Check sheet for the drawn part. Datum: minimum x, y, z corner. Units: mm. Coordinates: 2 decimals unless noted, no trailing zeros. Loops run counter-clockwise (first coordinate to the right, second up) from the corner with the lowest first, then second, coordinate; pieces in that order, holes last.
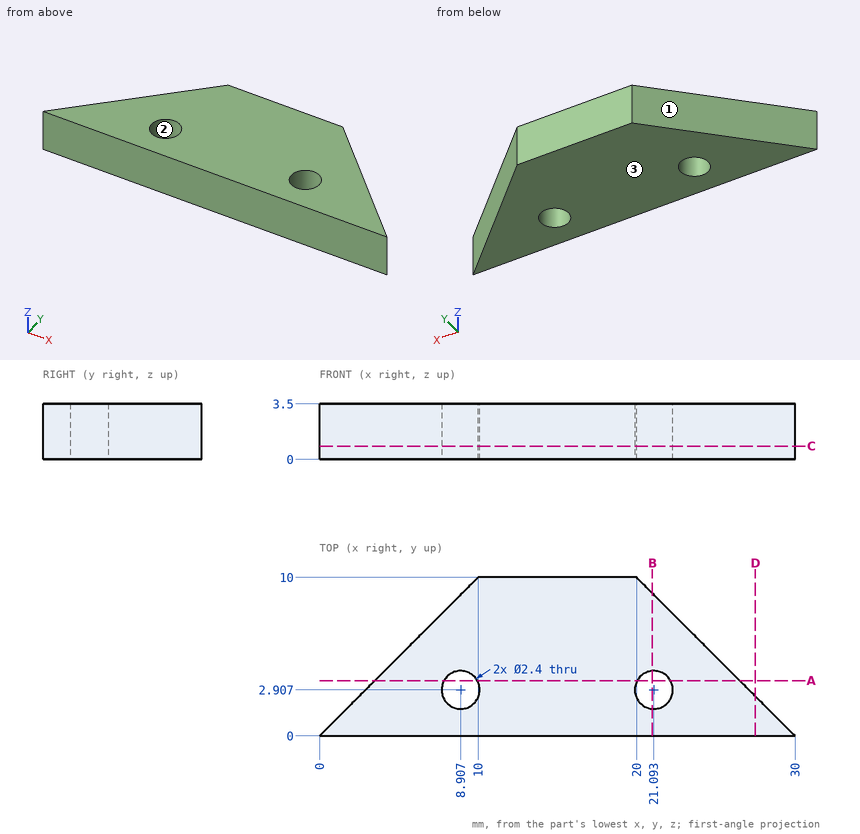
(1) Sectioned sample at D-D on x = 27.5. Record the cut outline in (y, z).
Findings:
outline: (0, 0) - (2.5, 0) - (2.5, 3.5) - (0, 3.5) - close
(2) Scan lines: L1, parallel to X at y = 2.25, z = 2.1; L2, parallel to Y at x = 8.5, z = 0.6 (1 decimal); L3, parallel to Y at x = 8, z = 1.4 (1 decimal). Record each from-to range of solid material in increasing order.
Findings:
L1: x = 2.25 to 7.9, 9.91 to 20.09, 22.1 to 27.75
L2: y = 0 to 1.8, 4 to 8.5
L3: y = 0 to 2.1, 3.7 to 8
(3) Draft check along X on the marked faces 1, 2 and 3. Enter one of: +X half, -X half, draft (parallel to the pull), parting line (faces both ways), or undercut.
Findings:
face 1: -X half
face 2: undercut
face 3: draft
(4) Sectioned sample at A-A on y = 3.5. Record the cut outline in (x, z).
Findings:
outline: (3.5, 0) - (7.86, 0) - (7.86, 3.5) - (3.5, 3.5) - close; (9.95, 0) - (20.05, 0) - (20.05, 3.5) - (9.95, 3.5) - close; (22.14, 0) - (26.5, 0) - (26.5, 3.5) - (22.14, 3.5) - close
(5) Sectioned sample at C-C on z = 0.85. Record the cut outline in (x, y), and give its area (3 significant figures).
Findings:
outline: (0, 0) - (30, 0) - (20, 10) - (10, 10) - close; hole circle Ø2.4 at (8.91, 2.91); hole circle Ø2.4 at (21.09, 2.91)
area: 191 mm2
(6) Sectioned sample at B-B on x = 21. Record the cut outline in (y, z).
Findings:
outline: (0, 0) - (1.71, 0) - (1.71, 3.5) - (0, 3.5) - close; (4.1, 0) - (9, 0) - (9, 3.5) - (4.1, 3.5) - close
(7) Gauge pin test, flat end, axial feed: pin 1 Ø1 at (y, z) = (5.5, 2) entering from -X. Record the tip position at first contact, or that the pin passes through.
Findings:
pin 1: stops at x = 5
